Input: part model. Units: mm. Frame: model coordinates. A direction names the side the tool comes from. Coordinates: 2 decimals unless noted, no trailing zeros. Order: outer loops, then holes, each group sorted by start corner. A loop starts at its lowest first (then second) coordinate and runs counter-clockwise, first axis right, second up.
from build123d import *

# Parameters (mm, degrees)
EXTRUDE_1_DEPTH     = 3
CUT_EXTRUDE_1_DEPTH = 10
FILLET_2_R          = 20
EXTRUDE_START       = 4.55
SKETCH_4_R          = 11
SKETCH_4_R_2        = 9
EXTRUDE_2_DEPTH     = 4.55
EXTRUDE_3_DEPTH     = 4.55


with BuildPart() as part:
    # 草图1 → 凸台-拉伸1 (new body)
    with BuildSketch(Plane.XY):
        with BuildLine():
            Line((-27.595006342, -7.125), (-10.650704202, -72.75))
            ThreePointArc((-10.650704202, -72.75), (0, -81), (10.650704202, -72.75))
            Line((10.650704202, -72.75), (27.595006342, -7.125))
            ThreePointArc((27.595006342, -7.125), (0, 28.5), (-27.595006342, -7.125))
        make_face()
    extrude(amount=EXTRUDE_1_DEPTH)

    # 草图2 → 切除-拉伸1 (cut)
    with BuildSketch(Plane.XY.offset(3)):
        Polygon((-12.872325689, -64.14569698), (-3.433026856, -37.146128717), (-28.154763001, -4.957071782), align=None)
    extrude(amount=-CUT_EXTRUDE_1_DEPTH, mode=Mode.SUBTRACT)

    # 圆角2
    fillet_2_edges = [part.edges().sort_by_distance(p)[0] for p in [
        (-12.872325689, -64.14569698, 1.5),
        (-28.03841186, -5.108567351, 1.5),
        (-3.433026856, -37.146128717, 1.5),
    ]]
    fillet(fillet_2_edges, radius=FILLET_2_R)

    # 草图4 → 凸台-拉伸2 (add)
    with BuildSketch(Plane(origin=(0, 0, 0), x_dir=(-1, 0, 0), z_dir=(0, 0, -1)).offset(EXTRUDE_START)):
        with Locations((0, -70)):
            Circle(SKETCH_4_R)
        with Locations((0, -70)):
            Circle(SKETCH_4_R_2, mode=Mode.SUBTRACT)
    extrude(amount=-EXTRUDE_2_DEPTH)

    # 草图5 → 凸台-拉伸3 (add)
    with BuildSketch(Plane(origin=(0, 0, 0), x_dir=(-1, 0, 0), z_dir=(0, 0, -1)).offset(EXTRUDE_START)):
        with BuildLine():
            Line((-10.650704202, -72.75), (-27.595006342, -7.125))
            ThreePointArc((-27.595006342, -7.125), (-6.884619071, 27.655958133), (27.714816001, 6.643716885))
            Line((27.714816001, 6.643716885), (25.769916632, 6.177491138))
            ThreePointArc((25.769916632, 6.177491138), (-6.401487908, 25.715189141), (-25.658514669, -6.625))
            Line((-25.658514669, -6.625), (-10.295351359, -66.126275643))
            ThreePointArc((-10.295351359, -66.126275643), (-10.984204203, -69.410713976), (-10.650704202, -72.75))
        make_face()
    extrude(amount=-EXTRUDE_3_DEPTH)


solid = part.part
Item 1: Cut plane D-D on x = -13. Return loops of the section in (y, z), then the cut area to 3 significant figures.
Response values:
outline: (-24.69, 0) - (23.09, 0) - (23.09, -4.55) - (25.36, -4.55) - (25.36, 3) - (-24.69, 3) - close
area: 160 mm2
Item 2: Access query for faces 4 (the face through (-26.756, 6.414, -2.307)), 5 (the face through (0, -70, 0)), 6 (the face through (0, -13, 3)). Directions: +Z, -Z, +X, -X, +Y, -Y. A direction counts if a zero-diameter tool reaches every point of the face in a straight line with its end or side. Return the directions, or none.
Response values:
face 4: -Z, -X, -Y
face 5: -Z
face 6: +Z, +X, -X, +Y, -Y
Item 3: Cut plane B-B on x = 0. Return loops of the section in (y, z).
Response values:
outline: (-81, -4.55) - (-79, -4.55) - (-79, 0) - (-61, 0) - (-61, -4.55) - (-59, -4.55) - (-59, 0) - (26.5, 0) - (26.5, -4.55) - (28.5, -4.55) - (28.5, 3) - (-81, 3) - close
Item 4: Cut plane C-C on y = 0. Return loops of the section in (x, z).
Response values:
outline: (-28.17, 0) - (26.5, 0) - (26.5, -4.55) - (28.5, -4.55) - (28.5, 3) - (-28.17, 3) - close
Item 5: Ray query, probe 1 along Y at (x, z) = (0, -1.2); probe 2 along Y at (x, z) = (-5, -4); probe 3 along Z at (x, y) = (-3, -24). Return the intervals inside material, ascending.
Response values:
probe 1: y = -81 to -79, -61 to -59, 26.5 to 28.5
probe 2: y = -79.8 to -77.48, -62.52 to -60.2, 26.02 to 28.06
probe 3: z = 0 to 3
Item 6: Pin query (flat end, axial travel): pin 1 Ø6 at (x, y) = (11.5, -10.5) entering from -Z; pin 2 Ø4 at (x, z) = (9.5, -1.5) entering from -Y; pin 3 Ø2 at (y, z) = (-53.5, 2) entering from +X. Return the tip coordinate at first contact, or that it passes through.
Response values:
pin 1: stops at z = 0
pin 2: stops at y = -78.05
pin 3: stops at x = 15.88
Item 7: Draft query along X for faces 1 (the face through (-8.96, -52.96, 1.52)), 2 (the face through (-1, -11, 0)), 3 (the face through (19.004, -40.397, -0.828)). Return one class per face: pulls with the +X half, pulls with the -X half, needs draft (parallel to the pull), parting line crosses it, or undercut.
Response values:
face 1: pulls with the -X half
face 2: undercut
face 3: pulls with the +X half
